The model under review builds one solid part; all positions refer to its coordinate system, in mm. Face numbers are marked on the shaded views. A direction names the side the tool comes from. Coordinates: 2 decimals unless noted, no trailing zeros. Write each loop counter-clockwise with the first axis right and the second up, starting at its lowest first coordinate (ties: lowest second). Pieces come first, ordered by that corner, then holes.
```python
from build123d import *

# Parameters (mm, degrees)
SKETCH1_R               = 6
SKETCH1_R_2             = 3.05
BOSS_EXTRUDE1_DEPTH     = 7.5
SKETCH2_R               = 10.5
BOSS_EXTRUDE3_DEPTH     = 18
BOSS_EXTRUDE4_DEPTH     = 18
CIRPATTERN1_COUNT       = 14
SKETCH3_R               = 3.05
CUT_EXTRUDE1_DEPTH      = 19
SKETCH5_W               = 1.3
SKETCH5_H               = 8.98796618
BOSS_EXTRUDE5_DEPTH     = 25.5
SKETCH4_R               = 1.4
CUT_EXTRUDE2_DEPTH      = 1
CUT_EXTRUDE2_DEPTH_BACK = 38.540546983


with BuildPart() as part:
    # Sketch1 → Boss-Extrude1 (new body)
    with BuildSketch(Plane.XY):
        with Locations((-24.192657344, -27.82930415)):
            Circle(SKETCH1_R)
        with Locations((-24.192657344, -27.82930415)):
            Circle(SKETCH1_R_2, mode=Mode.SUBTRACT)
    extrude(amount=BOSS_EXTRUDE1_DEPTH)

    # Sketch2 → Boss-Extrude3 (add)
    with BuildSketch(Plane.XY.offset(7.5)):
        with Locations((-24.192657344, -27.82930415)):
            Circle(SKETCH2_R)
    extrude(amount=BOSS_EXTRUDE3_DEPTH)

    # Sketch2<4> → Boss-Extrude4 (add)
    with BuildSketch(Plane.XY.offset(7.5)):
        with BuildLine():
            ThreePointArc((-22.692657344, -17.436999304), (-22.822516009, -15.882132595), (-23.192657344, -14.366392132))
            ThreePointArc((-23.192657344, -14.366392132), (-24.192657344, -14.32930415), (-25.192657344, -14.366392132))
            ThreePointArc((-25.192657344, -14.366392132), (-25.562798679, -15.882132595), (-25.692657344, -17.436999304))
            ThreePointArc((-25.692657344, -17.436999304), (-24.192657344, -17.32930415), (-22.692657344, -17.436999304))
        make_face()
    boss_extrude4 = extrude(amount=BOSS_EXTRUDE4_DEPTH)

    # CirPattern1: Boss-Extrude4 ×14 about axis
    cirpattern1_axis = Axis((-24.192657344, -27.82930415, 0), (0, 0, 1))
    for i in range(1, CIRPATTERN1_COUNT):
        add(boss_extrude4.rotate(cirpattern1_axis, i * 360 / CIRPATTERN1_COUNT))

    # Sketch3 → Cut-Extrude1 (cut, through all)
    with BuildSketch(Plane(origin=(0, 0, 7.5), x_dir=(-1, 0, 0), z_dir=(0, 0, -1))):
        with Locations((24.192657344, -27.82930415)):
            Circle(SKETCH3_R)
    extrude(amount=-CUT_EXTRUDE1_DEPTH, mode=Mode.SUBTRACT)

    # Sketch5 → Boss-Extrude5 (add, through all)
    with BuildSketch(Plane(origin=(0, 0, 0), x_dir=(-1, 0, 0), z_dir=(0, 0, -1))):
        with Locations((21.792657344, -27.156324883)):
            Rectangle(SKETCH5_W, SKETCH5_H)
    extrude(amount=-BOSS_EXTRUDE5_DEPTH)

    # Sketch4 → Cut-Extrude2 (cut, two sides)
    with BuildSketch(Plane(origin=(0, 0, 0), x_dir=(0, 0, -1), z_dir=(1, 0, 0))) as cut_extrude2_sk:
        with Locations((-3.5, -27.82930415)):
            Circle(SKETCH4_R)
    extrude(amount=CUT_EXTRUDE2_DEPTH, mode=Mode.SUBTRACT)
    extrude(cut_extrude2_sk.sketch, amount=-CUT_EXTRUDE2_DEPTH_BACK, mode=Mode.SUBTRACT)


solid = part.part
```
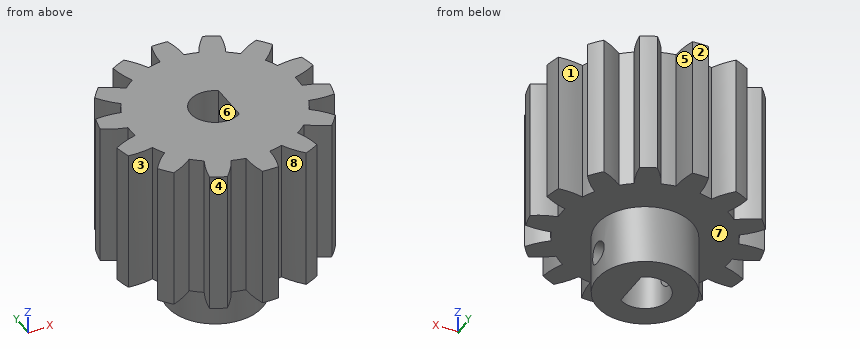
Item 1: Machinability: for the marked faces 5, 6, 7 and 8, which of the approach directions +Z, -Z, +X, -X, +Y, -Y give a long, thin tool a straight path to every point of the face, cutting with its end or side? Answer none if there is none.
Solved:
face 5: +Z, -Z, +Y
face 6: +Z, -Z
face 7: -Z
face 8: +Z, -Z, -Y
Item 2: To check wall thickness, follow line 1 along Y through (x, z) = (-13.25, 11); line 2 along Z through (x, y) = (-26.5, -20.75); line 3 along X through (y, z) = (-39.5, 20.25). State the ranges of each line that lie inside material, in increasing order.
Solved:
line 1: y = -35.74 to -35.14, -31.79 to -28.8, -26.86 to -23.87, -20.52 to -19.92
line 2: z = 7.5 to 25.5
line 3: x = -30.93 to -28.37, -25.6 to -22.78, -20.02 to -17.45
Item 3: Take a section at B-B, the plane z = 7. Write out the cut boundary in (x, y), plus the area to 3 significant figures.
Solved:
outline: circle Ø12 at (-24.19, -27.83); hole (-22.44, -30.33) - (-22.44, -25.33) arc R3.05 ccw (long way) to start
area: 88.4 mm2
Item 4: For pin 1 (2 mm diameter, centred on x = -33, z = 8, fed in from -Y); pin 2 (5 mm diameter, centred on y = -21.5, z = 8, fed in from +X); pin 3 (8 mm diameter, centred on x = -30.5, z = 18.5, fed in from +Y), all flat-tipped, find the tip position at first contact; note any pin that passes through.
Solved:
pin 1: stops at y = -36.97
pin 2: stops at x = -11.25
pin 3: stops at y = -15.27
Item 5: Mouldability with a two-part tool opening along Y and no side actions: class the marked faces 1, 2, 3 and 4 as pulls with the +Y half, pulls with the -Y half, needs draft (parallel to the pull), parting line crosses it, or undercut.
Solved:
face 1: undercut
face 2: pulls with the +Y half
face 3: undercut
face 4: pulls with the -Y half
Item 6: Take a section at A-A, the plane z = 3.5. Write out the cut boundary in (x, y), plus the area to 3 significant figures.
Solved:
outline: (-30.03, -29.23) arc R6 ccw to (-18.36, -29.23) - (-22.44, -29.23) - (-22.44, -30.33) arc R3.05 cw to (-26.9, -29.23) - close; (-30.03, -26.43) - (-26.9, -26.43) arc R3.05 cw to (-22.44, -25.33) - (-22.44, -26.43) - (-18.36, -26.43) arc R6 ccw to start
area: 68.3 mm2
